The listing builds one solid part. Answer for the finished solid, in the listing's coordinates (mm). Give positions to 0.01 mm unless a question says otherwise; leave off trailing zeros. Loops run counter-clockwise (first coordinate to the right, second up) from the corner with the lowest first, then second, coordinate; pieces in that order, holes last. Notation, with made-up numbers: M 64.25,-35 L 99.25,-35 A26 ccw 99.25,-16 Z; hole C 22,74.5 d10. An arc over 180 degrees is marked long. Use one line per item in the form item = value. Start each with the question number.
1. Each of these flat-tipped pins is pushed along its axis until it touches: pin 1 Ø5 at (x, z) = (89, 20) entering from +Y; pin 2 Ø10 at (y, z) = (35.5, 21) entering from -X; pin 3 Ø14 at (x, y) = (82.5, 26.5) entering from +Z. Where does it stop, or does it pass through?
2. The part is cut by section A-A (y = 0). Write down the section's boundary in (x, z), and give its area (3 significant figures).
3. The part is cut by section C-C (z = 25). Write down the section's boundary in (x, y).
4. Straight lines are drawn through the part: line 1 (Z direction, x = 73.5, y = 12.5); line 2 (Y direction, x = 60, z = 2.9); line 3 (Y direction, x = 91, z = 17.5). For each, find the intervals that lie inside material, in ascending order. Write a range as from..to.
5. The part is cut by section D-D (y = 25.5). Write down the section's boundary in (x, z).
6. The part is cut by section B-B (x = 92). Write down the section's boundary in (y, z), and give its area (3 significant figures).
7. The mould has two halves that part along X. Classify faces 1 (the face through (102.385, 0.751, 2.465)), 2 (the face through (85, 14, 0)), 3 (the face through (72.35, 23.03, 2.46)): released by +X, released by -X, zero draft, split by the parting line, or undercut.
from build123d import *

# Parameters (mm, degrees)
F0_R     = 2.5
F1_DEPTH = 5
F2_DEPTH = 50


with BuildPart() as f1:
    # F0 (on Top) → F1 (new body)
    with BuildSketch(Plane.XY):
        with BuildLine():
            Line((60, -5), (100, -5))
            ThreePointArc((100, -5), (103.872983, -3.162278), (104.898979, 1))
            Line((104.898979, 1), (96.898979, 40.191836))
            ThreePointArc((96.898979, 40.191836), (96.974681, 39.694381), (97, 39.191836))
            ThreePointArc((97, 39.191836), (90.321447, 34.48201), (88.127017, 42.354114))
            Line((88.127017, 42.354114), (56.127017, 3.162278))
            ThreePointArc((56.127017, 3.162278), (55.482734, -2.143433), (60, -5))
        make_face()
        with Locations((60, 0)):
            Circle(F0_R, mode=Mode.SUBTRACT)
        with Locations((100, 0)):
            Circle(F0_R, mode=Mode.SUBTRACT)
    extrude(amount=F1_DEPTH)

    # F0 (on Top) → F2 (join)
    with BuildSketch(Plane.XY):
        with BuildLine():
            ThreePointArc((97, 39.191836), (96.974681, 39.694381), (96.898979, 40.191836))
            ThreePointArc((96.898979, 40.191836), (93.196674, 44.046521), (88.127017, 42.354114))
            ThreePointArc((88.127017, 42.354114), (90.321447, 34.48201), (97, 39.191836))
        make_face()
    extrude(amount=F2_DEPTH)


solid = f1.part
Derived:
q1.pin_1 = 44.17
q1.pin_2 = 87
q1.pin_3 = 5
q2.outline = M 55,0 L 57.5,0 L 57.5,5 L 55,5 Z; M 62.5,0 L 97.5,0 L 97.5,5 L 62.5,5 Z; M 102.5,0 L 105,0 L 105,5 L 102.5,5 Z
q2.area = 200 mm2
q3.outline = M 96.9,40.19 A5 ccw long 97,39.19 A5 ccw Z
q4.line_1 = 0..5
q4.line_2 = -5..-2.5, 2.5..7.91
q4.line_3 = 34.29..44.09
q5.outline = M 74.37,0 L 99.9,0 L 99.9,5 L 74.37,5 Z
q6.outline = M -5,0 L 44.19,0 L 44.19,50 L 34.19,50 L 34.19,5 L -5,5 Z
q6.area = 696 mm2
q7.face_1 = undercut
q7.face_2 = zero draft
q7.face_3 = released by -X
